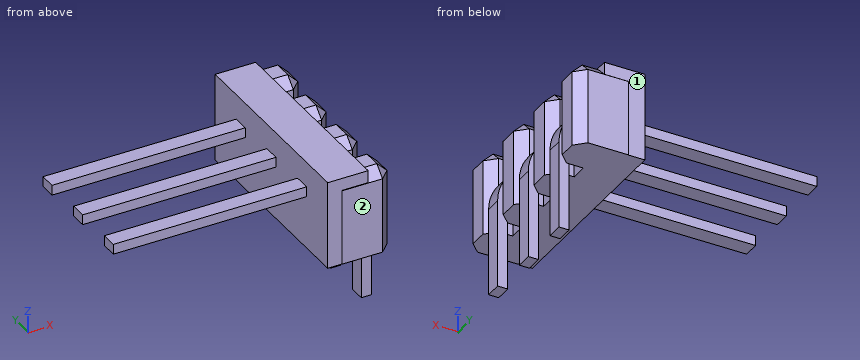
from build123d import *

# Parameters (mm, degrees)
BOX004_W                  = 1.6
BOX004_H                  = 8
BOX004_DEPTH              = 3.5
BOX003_W                  = 1.54
BOX003_H                  = 2
BOX003_DEPTH              = 3.4
CHAMFER002_SIZE           = 0.4
BOX002_W                  = 1.5
BOX002_H                  = 2
BOX002_DEPTH              = 3.4
CHAMFER001_SIZE           = 0.4
BOX_W                     = 1.54
BOX_H                     = 2
BOX_DEPTH                 = 3.4
CHAMFER003_SIZE           = 0.4
BOX001_W                  = 1.5
BOX001_H                  = 2
BOX001_DEPTH              = 3.4
CHAMFER_SIZE              = 0.4
SKETCH001_W               = 0.64
SKETCH001_H               = 0.4
ARRAY_X_COUNT             = 3
ARRAY_X_PITCH             = 2.18
FUSION001_PLACEMENT_ANGLE = -90


with BuildPart() as cubo008:
    # Box004 → Box004 (new body)
    with BuildSketch(Plane(origin=(-9.36, -4.13, 1.7), x_dir=(1, 0, 0), z_dir=(0, 0, 1))):
        with Locations((0.8, 4)):
            Rectangle(BOX004_W, BOX004_H)
    extrude(amount=BOX004_DEPTH)


with BuildPart() as chamfer002:
    # Box003 → Box003 (new body)
    with BuildSketch(Plane(origin=(-2.93, -3.3, 0.2), x_dir=(1, 0, 0), z_dir=(0, 0, 1))):
        with Locations((0.77, 1)):
            Rectangle(BOX003_W, BOX003_H)
    extrude(amount=BOX003_DEPTH)

    # Chamfer002
    chamfer002_edges = [chamfer002.edges().sort_by_distance(p)[0] for p in [
        (-2.93, -2.3, 3.6),
        (-2.93, -1.3, 1.9),
        (-1.39, -2.3, 3.6),
        (-1.39, -1.3, 1.9),
        (-2.16, -1.3, 3.6),
    ]]
    chamfer(chamfer002_edges, length=CHAMFER002_SIZE)


with BuildPart() as chamfer002_1:
    # Chamfer002 placement: moved
    add(chamfer002.part.moved(Location((3.2, 1.5, 1.5))))


with BuildPart() as chamfer001:
    # Box002 → Box002 (new body)
    with BuildSketch(Plane(origin=(-1.14, -16.5, 1.4), x_dir=(1, 0, 0), z_dir=(0, 0, 1))):
        with Locations((0.75, 1)):
            Rectangle(BOX002_W, BOX002_H)
    extrude(amount=BOX002_DEPTH)

    # Chamfer001
    chamfer001_edges = [chamfer001.edges().sort_by_distance(p)[0] for p in [
        (-1.14, -15.5, 4.8),
        (-1.14, -14.5, 3.1),
        (0.36, -15.5, 4.8),
        (0.36, -14.5, 3.1),
        (-0.39, -14.5, 4.8),
    ]]
    chamfer(chamfer001_edges, length=CHAMFER001_SIZE)


with BuildPart() as chamfer001_1:
    # Chamfer001 placement: moved
    add(chamfer001.part.moved(Location((5.78, 14.7, 0.3))))


with BuildPart() as chamfer003:
    # Box → Box (new body)
    with BuildSketch(Plane(origin=(-2.93, -3.3, 0.2), x_dir=(1, 0, 0), z_dir=(0, 0, 1))):
        with Locations((0.77, 1)):
            Rectangle(BOX_W, BOX_H)
    extrude(amount=BOX_DEPTH)

    # Chamfer003
    chamfer003_edges = [chamfer003.edges().sort_by_distance(p)[0] for p in [
        (-2.93, -2.3, 3.6),
        (-2.93, -1.3, 1.9),
        (-1.39, -2.3, 3.6),
        (-1.39, -1.3, 1.9),
        (-2.16, -1.3, 3.6),
    ]]
    chamfer(chamfer003_edges, length=CHAMFER003_SIZE)


with BuildPart() as chamfer003_1:
    # Chamfer003 placement: moved
    add(chamfer003.part.moved(Location((5.38, 1.5, 1.5))))


with BuildPart() as chamfer_body:
    # Box001 → Box001 (new body)
    with BuildSketch(Plane(origin=(-1.14, -16.5, 1.4), x_dir=(1, 0, 0), z_dir=(0, 0, 1))):
        with Locations((0.75, 1)):
            Rectangle(BOX001_W, BOX001_H)
    extrude(amount=BOX001_DEPTH)

    # Chamfer
    chamfer_edges = [chamfer_body.edges().sort_by_distance(p)[0] for p in [
        (-1.14, -15.5, 4.8),
        (-1.14, -14.5, 3.1),
        (0.36, -15.5, 4.8),
        (0.36, -14.5, 3.1),
        (-0.39, -14.5, 4.8),
    ]]
    chamfer(chamfer_edges, length=CHAMFER_SIZE)


with BuildPart() as chamfer_body_1:
    # Chamfer placement: moved
    add(chamfer_body.part.moved(Location((-0.74, 14.8, 0.3))))


with BuildPart() as obj1:
    # Sweep: sweep along a path in Sketch
    with BuildLine(Plane.YZ) as sweep_path:
        Line((0, 0), (0, 3.48702))
        ThreePointArc((0, 3.48702), (-0.443142, 4.556858), (-1.51298, 5))
        Line((-1.51298, 5), (-10, 5))
    # Sketch001 → Sweep (sweep)
    with BuildSketch(Plane.XY):
        Rectangle(SKETCH001_W, SKETCH001_H)
    sweep(path=sweep_path.line)


with BuildPart() as obj1_1:
    # Sweep placement: moved
    add(obj1.part.moved(Location((-0.05, 0, -1))))

    # Array X: obj1_3


with BuildPart() as obj1_2:
    add(obj1_1.part)
    with Locations(*[(i * ARRAY_X_PITCH, 0, 0) for i in range(1, ARRAY_X_COUNT)]):
        add(obj1_1.part)

    # Fusion001: union Chamfer002, Chamfer001, Chamfer003, Chamfer body
    add(chamfer002_1.part)
    add(chamfer001_1.part)
    add(chamfer003_1.part)
    add(chamfer_body_1.part)


with BuildPart() as obj1_3:
    # Fusion001 placement: moved
    add(obj1_2.part.moved(Location((-7, 2, 0))).rotate(Axis((-7, 2, 0), (0, 0, 1)), FUSION001_PLACEMENT_ANGLE))

    # Fusion: union Cubo008
    add(cubo008.part)


with BuildPart() as obj1_4:
    # Fusion placement: moved
    add(obj1_3.part.moved(Location((0, 2, 0))))


solid = obj1_4.part
Here's how the part is built. I have some questions about the finished solid (model axes, mm). Face numbers are marked on the shaded views. A direction names the side the tool comes from. Give positions to 0.01 mm unless a question says otherwise; leave off trailing zeros. Loops run counter-clockwise (first coordinate to the right, second up) from the corner with the lowest first, then second, coordinate; pieces in that order, holes last. Notation, with made-up numbers: (29.5, 75) -> (75.5, 75) arc R23 ccw to (75.5, 105) -> close; hole circle Ø9 at (12.25, -26.75). An arc over 180 degrees is marked (long way). One line per item, written item: value.
Q1. Suppose I cut it at A-A on z = 1.25. Please give me the cut outline in (x, y).
Answers follow:
outline: (-7.2, -0.63) -> (-6.8, -0.63) -> (-6.8, 0.01) -> (-7.2, 0.01) -> close; (-7.2, 1.55) -> (-6.8, 1.55) -> (-6.8, 2.19) -> (-7.2, 2.19) -> close; (-7.2, 3.73) -> (-6.8, 3.73) -> (-6.8, 4.37) -> (-7.2, 4.37) -> close
Q2. I'm going to push flat-ended pins straight in: pin 1 Ø3 at (x, y) = (-12.5, 2.5) entering from -Z; pin 2 Ø0.7 at (y, z) = (1.5, 2.5) entering from +X; pin 3 Ø1.5 at (y, z) = (4.5, 1) entering from -X. Where does each tip first touch, or does it pass through?
Answers follow:
pin 1: z = 3.8
pin 2: x = -6.8
pin 3: x = -9.36
Q3. Suppose I cut it at B-B on x = -10.5. Please give me the cut outline in (y, z), then the cut area to 3 significant figures.
Answers follow:
outline: (-0.63, 3.8) -> (0.01, 3.8) -> (0.01, 4.2) -> (-0.63, 4.2) -> close; (1.55, 3.8) -> (2.19, 3.8) -> (2.19, 4.2) -> (1.55, 4.2) -> close; (3.73, 3.8) -> (4.37, 3.8) -> (4.37, 4.2) -> (3.73, 4.2) -> close
area: 0.768 mm^2
Q4. Suppose I cut it at C-C on y = 3. Please give me the cut outline in (x, z), then the cut area to 3 significant figures.
Answers follow:
outline: (-9.36, 1.7) -> (-6.8, 1.7) -> (-6.8, 4.7) -> (-7.2, 5.1) -> (-7.76, 5.1) -> (-7.76, 5.2) -> (-9.36, 5.2) -> close
area: 8.78 mm^2
Q5. If I drill on line 1 along X through (y, z) = (2, 2.5); line 2 along Z through (x, y) = (-11, 4); line 3 along X through (y, z) = (5, 3.25), over which ranges is the centre line in solid material (lowest first)?
Answers follow:
line 1: -9.36 to -7.76, -7.2 to -6.8
line 2: 3.8 to 4.2
line 3: -9.36 to -6.7
Q6. On a 3-axis mill with a long thin cutter (end or side, diameter ignored), from which of +Z, -Z, +X, -X, +Y, -Y can I reach the whole of each face in a straight line? I mean the marked faces 1 and 2. Say none if no direction works.
Answers follow:
face 1: +Z, -X, +Y
face 2: +Z, -Z, +X, -X, -Y
